Can you work these out from the model? Positions are in its coordinate system, mm. A direction names the side the tool comes from. Give positions to 0.01 mm unless a question says otherwise; leave off trailing zeros. Write each loop counter-clockwise with the first axis right and the second up, starting at its lowest first coordinate (ties: lowest second). Pieces come first, ordered by that corner, then holes.
from build123d import *

# Parameters (mm, degrees)
SKETCH_2_W          = 50
SKETCH_2_H          = 7.55
SKETCH_2_R          = 1.6
EXTRUDE_1_DEPTH     = 4.9
SKETCH_3_W          = 24.132891974
SKETCH_3_H          = 13.680093874
SKETCH_3_R          = 1.6
EXTRUDE_2_DEPTH     = 10
SKETCH_4_W          = 10
SKETCH_4_H          = 10.264550668
CUT_EXTRUDE_1_DEPTH = 48.143107127
SKETCH_6_W          = 13.076103469
SKETCH_6_H          = 20.678046372
SKETCH_6_R          = 1.6
EXTRUDE_4_DEPTH     = 10
SKETCH_7_W          = 8
SKETCH_7_H          = 20.678046372
CUT_EXTRUDE_2_DEPTH = 10
EXTRUDE_5_DEPTH     = 10
SKETCH_9_W          = 12.029023446
SKETCH_9_H          = 8.2346335
SKETCH_9_W_2        = 7.42731649
SKETCH_9_H_2        = 3.390731441
CUT_EXTRUDE_3_DEPTH = 76.878053489


with BuildPart() as part:
    # Sketch 2 → Extrude 1 (new, symmetric)
    with BuildSketch(Plane(origin=(0, 0, 0), x_dir=(0, 0, -1), z_dir=(1, 0, 0))):
        with Locations((19.75, 0)):
            Rectangle(SKETCH_2_W, SKETCH_2_H)
        Circle(SKETCH_2_R, mode=Mode.SUBTRACT)
        with Locations((7, 0)):
            Circle(SKETCH_2_R, mode=Mode.SUBTRACT)
        with Locations((32.5, 0)):
            Circle(SKETCH_2_R, mode=Mode.SUBTRACT)
        with Locations((39.5, 0)):
            Circle(SKETCH_2_R, mode=Mode.SUBTRACT)
    extrude(amount=EXTRUDE_1_DEPTH, both=True)

    # Sketch 3 → Extrude 2 (add, symmetric)
    with BuildSketch(Plane(origin=(0, 0, 0), x_dir=(0, 0, -1), z_dir=(1, 0, 0))):
        with Locations((14.180871083, 10.615046937)):
            Rectangle(SKETCH_3_W, SKETCH_3_H)
        with Locations((7, 13)):
            Circle(SKETCH_3_R, mode=Mode.SUBTRACT)
        with Locations((20.26, 13)):
            Circle(SKETCH_3_R, mode=Mode.SUBTRACT)
    extrude(amount=EXTRUDE_2_DEPTH, both=True)

    # Sketch 4 → Cut-Extrude 1 (cut, through all)
    with BuildSketch(Plane.XY.offset(-2.114425096)):
        with Locations((0, 12.32281854)):
            Rectangle(SKETCH_4_W, SKETCH_4_H)
    extrude(amount=-CUT_EXTRUDE_1_DEPTH, mode=Mode.SUBTRACT)



with BuildPart() as body_2:
    # Sketch 6 → Extrude 4 (new, symmetric)
    with BuildSketch(Plane(origin=(0, 0, 0), x_dir=(0, 0, -1), z_dir=(1, 0, 0))):
        with Locations((64.164086861, 8.6)):
            Rectangle(SKETCH_6_W, SKETCH_6_H)
        with Locations((66.5, 3.6)):
            Circle(SKETCH_6_R, mode=Mode.SUBTRACT)
        with Locations((66.5, 13.6)):
            Circle(SKETCH_6_R, mode=Mode.SUBTRACT)
    extrude(amount=EXTRUDE_4_DEPTH, both=True)

    # Sketch 7 → Cut-Extrude 2 (cut)
    with BuildSketch(Plane.XY.offset(-70.702138596)):
        with Locations((0, 8.6)):
            Rectangle(SKETCH_7_W, SKETCH_7_H)
    extrude(amount=CUT_EXTRUDE_2_DEPTH, mode=Mode.SUBTRACT)


with BuildPart() as part_1:
    add(part.part)

    add(body_2.part)  # Extrude 5 merges body 2
    # Sketch 8 → Extrude 5 (add, symmetric)
    with BuildSketch(Plane(origin=(0, 0, 0), x_dir=(0, 0, -1), z_dir=(1, 0, 0))):
        Polygon((57.626035127, 18.939023186), (26.24731707, 18.939023186), (26.24731707, 11.139938787), (26.24731707, 3.775), (44.75, 3.775), (44.75, 11.139938787), (57.626035127, 11.139938787), align=None)
    extrude(amount=EXTRUDE_5_DEPTH, both=True)

    # Sketch 9 → Cut-Extrude 3 (cut, through all)
    with BuildSketch(Plane(origin=(10, 0, 0), x_dir=(0, 0, -1), z_dir=(1, 0, 0))):
        with Locations((35.100955195, 11.220670488)):
            Rectangle(SKETCH_9_W, SKETCH_9_H)
        with Locations((51.16656369, 15.337987238)):
            Rectangle(SKETCH_9_W_2, SKETCH_9_H_2)
    extrude(amount=-CUT_EXTRUDE_3_DEPTH, mode=Mode.SUBTRACT)


solid = part_1.part
(1) Imagine slicing it at D-D, the plane z = -39.5. Write out the boundary of the cut face in (x, y) (3 decimals), plus the area to 3 significant figures.
Returned:
outline: (-10, 3.775) - (-4.9, 3.775) - (-4.9, 1.6) - (4.9, 1.6) - (4.9, 3.775) - (10, 3.775) - (10, 7.103) - (-10, 7.103) - close; (-10, 15.338) - (10, 15.338) - (10, 18.939) - (-10, 18.939) - close; (-4.9, -3.775) - (4.9, -3.775) - (4.9, -1.6) - (-4.9, -1.6) - close
area: 181 mm2
(2) Imagine slicing it at C-C, the plane x = -3.25. Write out the boundary of the cut face in (y, z) (3 decimals).
Returned:
outline: (-3.775, -44.75) - (11.14, -44.75) - (11.14, -57.626) - (-1.739, -57.626) - (-1.739, -60.702) - (18.939, -60.702) - (18.939, -26.247) - (7.191, -26.247) - (7.191, -2.114) - (3.775, -2.114) - (3.775, 5.25) - (-3.775, 5.25) - close; hole circle Ø3.2 at (0, -39.5); hole circle Ø3.2 at (0, -32.5); hole circle Ø3.2 at (0, -7); hole circle Ø3.2 at (0, 0); hole (7.103, -41.115) - (15.338, -41.115) - (15.338, -29.086) - (7.103, -29.086) - close; hole (13.643, -54.88) - (17.033, -54.88) - (17.033, -47.453) - (13.643, -47.453) - close
(3) Will these pins go through, and if not, where does the flat tip stop? P1, Ø8, axis at y = 8.5, z = -55.5, coming from the -X side; P2, Ø4, axis at y = 0, z = -7, coming from the -X side; P3, Ø1.9, axis at y = 13, z = -20.26, coming from the -X side; P4, Ø4, axis at x = 7.5, z = -17.5, coming from the +Y side.
Returned:
P1: stops at x = -10
P2: stops at x = -4.9
P3: passes through
P4: stops at y = 17.46
(4) Imagine slicing it at B-B, the plane y = 6. Write out the boundary of the cut face in (x, z), plus the area to 3 significant figures.
Returned:
outline: (-10, -70.7) - (-4, -70.7) - (-4, -60.7) - (4, -60.7) - (4, -70.7) - (10, -70.7) - (10, -57.63) - (-10, -57.63) - close; (-10, -44.75) - (10, -44.75) - (10, -2.11) - (-10, -2.11) - close
area: 1,030 mm2
(5) Imagine slicing it at A-A, the plane z = -7. Write out the boundary of the cut face in (x, y) (3 decimals), plus the area to 3 significant figures.
Returned:
outline: (-10, 3.775) - (-4.9, 3.775) - (-4.9, 1.6) - (4.9, 1.6) - (4.9, 3.775) - (10, 3.775) - (10, 11.4) - (5, 11.4) - (5, 7.191) - (-5, 7.191) - (-5, 11.4) - (-10, 11.4) - close; (-10, 14.6) - (-5, 14.6) - (-5, 17.455) - (-10, 17.455) - close; (-4.9, -3.775) - (4.9, -3.775) - (4.9, -1.6) - (-4.9, -1.6) - close; (5, 14.6) - (10, 14.6) - (10, 17.455) - (5, 17.455) - close
area: 182 mm2
(6) If I drill on L1, parallel to Y at x = -7.3, z = -66.5; L2, parallel to Y at x = 8.3, z = -7 (3 decimals); L3, parallel to Z at x = -1.5, y = 7.5, over which ranges is the centre line in solid material (lowest first)?
Returned:
L1: y = -1.74 to 2, 5.2 to 12, 15.2 to 18.94
L2: y = 3.775 to 11.4, 14.6 to 17.455
L3: z = -60.7 to -57.63, -44.75 to -41.12, -29.09 to -26.25
(7) If we mould it in two halves opening along Y, with no side actions, what happens to faces 1 (the face through (0, 5, -57.626)), 2 (the face through (0, -1.739, -60)), 3 (the face through (7.5, 14.1, -19.1))? For each: +Y half, -Y half, draft (parallel to the pull), parting line (faces both ways), or undercut.
Returned:
face 1: draft
face 2: -Y half
face 3: undercut
(8) For faces 4 (the face through (0, 6, -2.114)), 5 (the face through (-7, 3.775, -23)), 6 (the face through (0, 11.14, -51)), which set-ups out of +Z, -Z, +X, -X, +Y, -Y let a thin tool reach every point of the face, with its end or its side?
Returned:
face 4: +Z, +X, -X, +Y
face 5: +Z, -X, -Y
face 6: +X, -X, -Y
